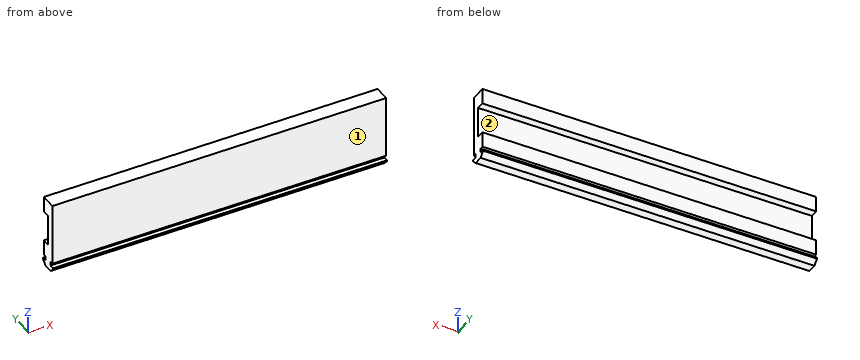
from build123d import *

# Parameters (mm, degrees)
SKETCH1_R           = 2.1
BOSS_EXTRUDE1_DEPTH = 65
SKETCH84_W          = 0.3
SKETCH84_H          = 5.4
BOSS_EXTRUDE6_DEPTH = 430
SKETCH85_W          = 26.589814492
SKETCH85_H          = 26.977421118
CUT_EXTRUDE59_DEPTH = 434.070721707
SKETCH86_W          = 10.5
SKETCH86_H          = 16.670499862
CUT_EXTRUDE60_DEPTH = 20
SKETCH87_W          = 62.679537103
SKETCH87_H          = 29.503453987
CUT_EXTRUDE61_DEPTH = 215
BOSS_EXTRUDE7_DEPTH = 215


with BuildPart() as part:
    # Sketch1 → Boss-Extrude1 (new body)
    with BuildSketch(Plane(origin=(0, 0, 0), x_dir=(0, 0, -1), z_dir=(1, 0, 0))):
        with BuildLine():
            Line((-10, 9), (-10, 3))
            Line((-10, 3), (-8, 3))
            Line((-8, 3), (-8, 6))
            Line((-8, 6), (-7.060660172, 6))
            Line((-7.060660172, 6), (-4, 2.939339828))
            Line((-4, 2.939339828), (-4, -2.939339828))
            Line((-4, -2.939339828), (-7.060660172, -6))
            Line((-7.060660172, -6), (-8, -6))
            Line((-8, -6), (-8, -3))
            Line((-8, -3), (-10, -3))
            Line((-10, -3), (-10, -9))
            ThreePointArc((-10, -9), (-9.707106781, -9.707106781), (-9, -10))
            Line((-9, -10), (-3, -10))
            Line((-3, -10), (-3, -8))
            Line((-3, -8), (-6, -8))
            Line((-6, -8), (-6, -7.060660172))
            Line((-6, -7.060660172), (-2.939339828, -4))
            Line((-2.939339828, -4), (2.939339828, -4))
            Line((2.939339828, -4), (6, -7.060660172))
            Line((6, -7.060660172), (6, -8))
            Line((6, -8), (3, -8))
            Line((3, -8), (3, -10))
            Line((3, -10), (9, -10))
            ThreePointArc((9, -10), (9.707106781, -9.707106781), (10, -9))
            Line((10, -9), (10, -3))
            Line((10, -3), (8, -3))
            Line((8, -3), (8, -6))
            Line((8, -6), (7.060660172, -6))
            Line((7.060660172, -6), (4, -2.939339828))
            Line((4, -2.939339828), (4, 2.939339828))
            Line((4, 2.939339828), (7.060660172, 6))
            Line((7.060660172, 6), (8, 6))
            Line((8, 6), (8, 3))
            Line((8, 3), (10, 3))
            Line((10, 3), (10, 9))
            ThreePointArc((10, 9), (9.707106781, 9.707106781), (9, 10))
            Line((9, 10), (3, 10))
            Line((3, 10), (3, 8))
            Line((3, 8), (6, 8))
            Line((6, 8), (6, 7.060660172))
            Line((6, 7.060660172), (2.939339828, 4))
            Line((2.939339828, 4), (-2.939339828, 4))
            Line((-2.939339828, 4), (-6, 7.060660172))
            Line((-6, 7.060660172), (-6, 8))
            Line((-6, 8), (-3, 8))
            Line((-3, 8), (-3, 10))
            Line((-3, 10), (-9, 10))
            ThreePointArc((-9, 10), (-9.707106781, 9.707106781), (-10, 9))
        make_face()
        Circle(SKETCH1_R, mode=Mode.SUBTRACT)
    extrude(amount=BOSS_EXTRUDE1_DEPTH)

    # Sketch85 → Cut-Extrude59 (cut, through all)
    with BuildSketch(Plane(origin=(65, 0, 0), x_dir=(0, 0, -1), z_dir=(1, 0, 0))):
        with Locations((1.176321583, -0.814927094)):
            Rectangle(SKETCH85_W, SKETCH85_H)
    extrude(amount=-CUT_EXTRUDE59_DEPTH, mode=Mode.SUBTRACT)


with BuildPart() as body_2:
    # Sketch84 → Boss-Extrude6 (new body)
    with BuildSketch(Plane(origin=(65, 0, 0), x_dir=(0, 0, -1), z_dir=(1, 0, 0))):
        Polygon((-10, -2.7), (-10, 2.7), (-10.5, 2.7), (-10.5, 5), (-20.5, 5), (-20.5, 0), (-40.5, 0), (-40.5, 5), (-50.5, 5), (-50.5, -5), (-10.5, -5), (-10.5, -2.7), align=None)
        Polygon((-7.18492424, 5.7), (-4.3, 2.81507576), (-4.3, -2.81507576), (-7.18492424, -5.7), (-7.7, -5.7), (-7.7, -2.7), (-9.7, -2.7), (-9.7, 2.7), (-7.7, 2.7), (-7.7, 5.7), align=None)
        with Locations((-9.85, 0)):
            Rectangle(SKETCH84_W, SKETCH84_H)
    extrude(amount=BOSS_EXTRUDE6_DEPTH)

    # Sketch86 → Cut-Extrude60 (cut)
    with BuildSketch(Plane.ZY.offset(-65)):
        with Locations((5.25, -0.117074477)):
            Rectangle(SKETCH86_W, SKETCH86_H)
    extrude(amount=-CUT_EXTRUDE60_DEPTH, mode=Mode.SUBTRACT)

    # Sketch87 → Cut-Extrude61 (cut)
    with BuildSketch(Plane.ZY.offset(-65)):
        with Locations((27.544038236, 0.275447184)):
            Rectangle(SKETCH87_W, SKETCH87_H)
    extrude(amount=-CUT_EXTRUDE61_DEPTH, mode=Mode.SUBTRACT)

    # Sketch88 → Boss-Extrude7 (add)
    with BuildSketch(Plane.ZY.offset(-280)):
        Polygon((10.7, 2.9), (10.7, -2.9), (7.9, -2.9), (7.9, -5.9), (7.102081528, -5.9), (4.1, -2.897918472), (4.1, 2.897918472), (7.102081528, 5.9), (7.9, 5.9), (7.9, 2.9), align=None)
        Polygon((10.5, 2.7), (10.5, -2.7), (7.7, -2.7), (7.7, -5.7), (7.18492424, -5.7), (4.3, -2.81507576), (4.3, 2.81507576), (7.18492424, 5.7), (7.7, 5.7), (7.7, 2.7), align=None, mode=Mode.SUBTRACT)
    extrude(amount=-BOSS_EXTRUDE7_DEPTH)


solid = body_2.part
Input: part model. Units: mm. Frame: model coordinates. Face numbers are marked on the shaded views. Coordinates: 2 decimals unless noted, no trailing zeros. Loops run counter-clockwise (first coordinate to the right, second up) from the corner with the lowest first, then second, coordinate; pieces in that order, holes last. Notation, with made-up numbers: (71.25, -27) - (112.25, -27) arc R18 cw to (112.25, -6) - close; hole circle Ø1 at (-2, 60.25). An arc over 180 degrees is marked (long way). Answer in a Markdown table with one row per item. Add a question column.
Item 1: Line query: line 1 along Z through (x, y) = (432, 2.75); line 2 along Y through (x, z) = (477.5, 41); line 3 along Z through (x, y) = (305.5, 4). Output: solid intervals per line, ascending. Write a range as [from, to].
Item 2: Section query A-A on x = 422. Return the cut outline in (y, z).
Item 3: Mould query, pull axis Z, two halves, no side actions, for the marked faces 1 and 2. Classes: released by +Z, released by -Z, zero draft, split by the parting line, or undercut.
Item 4: Section query B-B on z = 18.5. Return the cut outline in (x, y).
Item 5: Contact query for flat-ended pins moving along their axis: P1, Ø3, axis at x = 364.5, z = 43.5, coming from the +Y side; P2, Ø0.8, axis at x = 336, z = 9, coming from the -Y side; P3, Ø1.7, axis at x = 394.5, y = 4, coming from the -Z side. Output: stop coordinate, or through.
Recorded:
| question | item | result |
|---|---|---|
| 1 | line 1 | [4.1, 20.5], [40.5, 50.5] |
| 1 | line 2 | [-5, 5] |
| 1 | line 3 | [5.2, 7.9], [10.5, 20.5], [40.5, 50.5] |
| 2 | outline | (-5.9, 7.1) - (-2.9, 4.1) - (2.9, 4.1) - (5.9, 7.1) - (5.9, 7.9) - (2.9, 7.9) - (2.9, 10.5) - (5, 10.5) - (5, 20.5) - (0, 20.5) - (0, 40.5) - (5, 40.5) - (5, 50.5) - (-5, 50.5) - (-5, 10.5) - (-2.9, 10.5) - (-2.9, 7.9) - (-5.9, 7.9) - close |
| 3 | face 1 | zero draft |
| 3 | face 2 | undercut |
| 4 | outline | (280, -5) - (495, -5) - (495, 5) - (280, 5) - close |
| 5 | P1 | y = 5 |
| 5 | P2 | y = -2.9 |
| 5 | P3 | z = 4.35 |
